Read the model definition and answer for the solid it produces. Units are mm, in the model's axes. Face numbers are marked on the shaded views. Give positions to 0.01 mm unless a question says otherwise; leave off trailing zeros. Loops run counter-clockwise (first coordinate to the right, second up) from the corner with the lowest first, then second, coordinate; pieces in that order, holes last.
(1) Determine the mould class of the marked faces 1 and 2 for opening direction Y: pulls with the +Y half, pulls with the -Y half, needs draft (parallel to the pull), parting line crosses it, or undercut.
(2) Find section A-A, the plane z = 41.5. Write down the section's boundary in (x, y).
(3) Each of these flat-tipped pins is pushed along its axis until it touches: P1, Ø10, axis at x = -52, y = -21.5, coming from the -Z side; P2, Ø16, axis at x = -138.5, z = -131.5, coming from the +Y side; P3, Ø6, axis at y = 144.5, z = -258, coming from the -X side. Where does it stop, or does it pass through?
(4) Straight lines are drawn through the part: probe 1 along Z at (x, y) = (-92, -1.5); probe 2 along Z at (x, y) = (135, 140.5). For each, find the intervals that lie inside material, in ascending order.
(5) Find section B-B, the plane x = 101. Write down the section's boundary in (y, z).
(6) Find section C-C, the plane z = -178.5. Write down the section's boundary in (x, y).
(7) Find section D-D, the plane y = -74. Write down the section's boundary in (x, z).
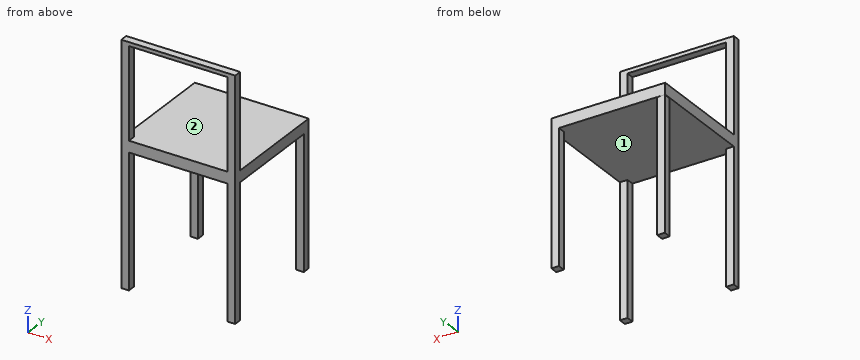
```python
from build123d import *

# Parameters (mm, degrees)
F0_W     = 300
F0_H     = 300
F1_DEPTH = 30
F3_W     = 20
F3_H     = 20
F4_DEPTH = 350
F5_W     = 20
F5_H     = 20
F6_DEPTH = 250
F7_W     = 20
F7_H     = 10
F8_DEPTH = 260


with BuildPart() as f1:
    # F0 (on Top) → F1 (new body)
    with BuildSketch(Plane.XY):
        with Locations((0.250861, 3.03171)):
            Rectangle(F0_W, F0_H)
    extrude(amount=F1_DEPTH)

    # F3 (on face) → F4 (join)
    with BuildSketch(Plane(origin=(0, 0, 0), x_dir=(1, 0, 0), z_dir=(0, 0, -1))):
        with Locations((-138.477522, -142.692491)):
            Rectangle(F3_W, F3_H)
        with Locations((-139.749139, 136.96829)):
            Rectangle(F3_W, F3_H)
        with Locations((140.250861, -143.03171)):
            Rectangle(F3_W, F3_H)
        with Locations((140.250861, 136.96829)):
            Rectangle(F3_W, F3_H)
    extrude(amount=F4_DEPTH)

    # F5 (on face) → F6 (join)
    with BuildSketch(Plane.XY.offset(30)):
        with Locations((140.250861, -136.96829)):
            Rectangle(F5_W, F5_H)
        with Locations((-139.749139, -136.96829)):
            Rectangle(F5_W, F5_H)
    extrude(amount=F6_DEPTH)

    # F7 (on face) → F8 (join)
    with BuildSketch(Plane(origin=(130.250861, 0, 0), x_dir=(0, -1, 0), z_dir=(-1, 0, 0))):
        with Locations((136.96829, 275)):
            Rectangle(F7_W, F7_H)
    extrude(amount=F8_DEPTH)


solid = f1.part
```
Entries:
1. face 1: undercut
1. face 2: needs draft
2. outline: (-149.75, -146.97) - (-129.75, -146.97) - (-129.75, -126.97) - (-149.75, -126.97) - close; (130.25, -146.97) - (150.25, -146.97) - (150.25, -126.97) - (130.25, -126.97) - close
3. P1: stops at z = 0
3. P2: stops at y = 152.69
3. P3: stops at x = -148.48
4. probe 1: z = 0 to 30
4. probe 2: z = -350 to 30
5. outline: (-146.97, 0) - (153.03, 0) - (153.03, 30) - (-146.97, 30) - close; (-146.97, 270) - (-126.97, 270) - (-126.97, 280) - (-146.97, 280) - close
6. outline: (-149.75, -146.97) - (-129.75, -146.97) - (-129.75, -126.97) - (-149.75, -126.97) - close; (-148.48, 132.69) - (-128.48, 132.69) - (-128.48, 152.69) - (-148.48, 152.69) - close; (130.25, -146.97) - (150.25, -146.97) - (150.25, -126.97) - (130.25, -126.97) - close; (130.25, 133.03) - (150.25, 133.03) - (150.25, 153.03) - (130.25, 153.03) - close
7. outline: (-149.75, 0) - (150.25, 0) - (150.25, 30) - (-149.75, 30) - close
